Solid Edge part; units mm, degrees
sketch "Sketch1" plane through (0, 0, 0) normal (0, 0, 1) x (1, 0, 0)
  line L0 (16.45, -16.45) -> (-16.45, -16.45)
  line L1 (-16.45, -16.45) -> (-16.45, 16.45)
  line L2 (-16.45, 16.45) -> (16.45, 16.45)
  line L3 (16.45, 16.45) -> (16.45, -16.45)
extrude "Protrusion1" add sketch "Sketch1" along normal blind 24.7
sketch "Sketch2" plane through (0, 0, 24.7) normal (0, 0, 1) x (1, 0, 0)
  circle A0 centre (-14, 14) radius 0.35
  circle A1 centre (14, 14) radius 0.85
  circle A2 centre (-14, -14) radius 0.85
  circle A3 centre (14, -14) radius 0.35
extrude "ExtrudedCutout_1" cut sketch "Sketch2" against normal blind 2
sketch "Sketch3" plane through (0, 0, 24.7) normal (0, 0, 1) x (1, 0, 0)
  circle A0 centre (0, 0) radius 0.95
extrude "ExtrudedProtrusion_2" add sketch "Sketch3" along normal blind 30
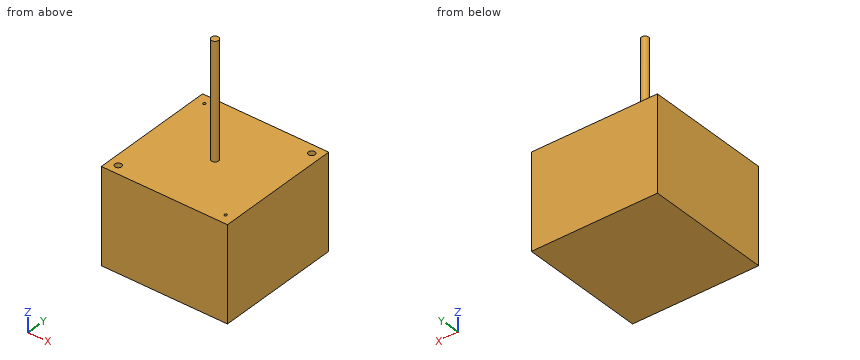
Here's how the part is built. I have some questions about the finished solid (model axes, mm). Coordinates: 2 decimals unless noted, no trailing zeros. Order: outer loops, then holes, each group sorted by start corner. A loop starts at its lowest first (then second) coordinate and runs counter-clockwise, first axis right, second up.
1) Will these pins go through, and if not, where does the flat tip stop? pin 1 (4 mm diameter, centred on x = -13, y = 4.5, fed in from +Z); pin 2 (1.5 mm diameter, centred on x = -14, y = -14, fed in from +Z); pin 3 (4 mm diameter, centred on y = 2.5, z = 38.5, fed in from +X); pin 4 (16.5 mm diameter, centred on x = -1.5, y = 1.5, fed in from +Z).
2) Imagine slicing it at B-B on x = -5. List the corners of the cut face in (y, z) for me, and give its area (3 significant figures).
3) I need wall thicknesses on line 1 (Y direction, x = -14, z = 23); line 2 (Y direction, x = 14, z = 24); line 3 (Z direction, x = -13, y = 4). Which ranges of each line are inside material? Lowest first, please.
4) Imagine slicing it at A-A on y = 0. List the corners of the cut face in (x, z) for me.
5) Imagine slicing it at C-C on z = 39.5. List the corners of the cut face in (x, y) for me, and give its area (3 significant figures).
Response values:
1. pin 1: stops at z = 24.7
1. pin 2: stops at z = 22.7
1. pin 3: stops at x = 0.81
1. pin 4: stops at z = 54.7
2. outline: (-16.45, 0) - (16.45, 0) - (16.45, 24.7) - (-16.45, 24.7) - close
2. area: 813 mm2
3. line 1: y = -16.45 to -14.85, -13.15 to 13.65, 14.35 to 16.45
3. line 2: y = -16.45 to -14.35, -13.65 to 13.15, 14.85 to 16.45
3. line 3: z = 0 to 24.7
4. outline: (-16.45, 0) - (16.45, 0) - (16.45, 24.7) - (0.95, 24.7) - (0.95, 54.7) - (-0.95, 54.7) - (-0.95, 24.7) - (-16.45, 24.7) - close
5. outline: circle Ø1.9 at (0, 0)
5. area: 2.84 mm2
